Check sheet for the modelled part. Datum: model origin and axes. Units: mm. Face numbers are marked on the shaded views. Round coordinates to 2 decimals unless told otherwise and drop trailing zeros. Write each loop counter-clockwise with the first axis right and the second up, starting at its lowest first coordinate (ties: lowest second). Pieces come first, ordered by that corner, then holes. Notation, with made-up numbers: M 67,4.5 L 122,4.5 A28 ccw 122,35.5 Z; hole C 80.5,65 d7. An arc over 180 degrees is marked long. One line per item, written item: value.
from build123d import *

# Parameters (mm, degrees)
F1_DEPTH = 100
F2_R     = 7.5
F3_DEPTH = 10
F4_R     = 4
F6_DEPTH = 25


with BuildPart() as f1:
    # F0 (on Top) → F1 (new body)
    with BuildSketch(Plane.XY):
        Polygon((25.9807621135, -45), (25.9807621135, 45), (-51.9615242271, 0), align=None)
    extrude(amount=F1_DEPTH)

    # F2 (on face) → F3 (cut)
    with BuildSketch(Plane.YZ.offset(25.9807621135)):
        with Locations((-30, 80)):
            Circle(F2_R)
        with Locations((30, 80)):
            Circle(F2_R)
    extrude(amount=-F3_DEPTH, mode=Mode.SUBTRACT)

    # F4
    f4_edges = [f1.edges().sort_by_distance(p)[0] for p in [
        (25.980762, -45, 50),
        (25.980762, 45, 50),
        (-51.961524, 0, 50),
        (-12.990381, -22.5, 100),
        (-12.990381, 22.5, 100),
        (25.980762, 0, 100),
        (-12.990381, -22.5, 0),
        (25.980762, 0, 0),
        (-12.990381, 22.5, 0),
    ]]
    fillet(f4_edges, radius=F4_R)

    # F5 (on face) → F6 (cut)
    with BuildSketch(Plane(origin=(0, 0, 0), x_dir=(1, 0, 0), z_dir=(0, 0, -1))):
        with BuildLine():
            Line((12.2403810568, -21.2009618943), (9.7403810568, -16.8708348754))
            ThreePointArc((9.7403810568, -16.8708348754), (8.8253175473, -20.2858983849), (12.2403810568, -21.2009618943))
        make_face()
        with BuildLine():
            ThreePointArc((13.4903810568, -19.0358983849), (12.2403810568, -16.8708348754), (9.7403810568, -16.8708348754))
            Line((9.7403810568, -16.8708348754), (12.2403810568, -21.2009618943))
            ThreePointArc((12.2403810568, -21.2009618943), (13.1554445662, -20.2858983849), (13.4903810568, -19.0358983849))
        make_face()
        with BuildLine():
            ThreePointArc((-24.4807621135, 0), (-21.9807621135, -2.5), (-19.4807621135, 0))
            Line((-19.4807621135, 0), (-24.4807621135, 0))
        make_face()
        with BuildLine():
            Line((-24.4807621135, 0), (-19.4807621135, 0))
            ThreePointArc((-19.4807621135, 0), (-21.9807621135, 2.5), (-24.4807621135, 0))
        make_face()
        with BuildLine():
            ThreePointArc((12.2403810568, 21.2009618943), (8.8253175473, 20.2858983849), (9.7403810568, 16.8708348754))
            Line((9.7403810568, 16.8708348754), (12.2403810568, 21.2009618943))
        make_face()
        with BuildLine():
            Line((12.2403810568, 21.2009618943), (9.7403810568, 16.8708348754))
            ThreePointArc((9.7403810568, 16.8708348754), (12.2403810568, 16.8708348754), (13.4903810568, 19.0358983849))
            ThreePointArc((13.4903810568, 19.0358983849), (13.1554445662, 20.2858983849), (12.2403810568, 21.2009618943))
        make_face()
    extrude(amount=-F6_DEPTH, mode=Mode.SUBTRACT)


solid = f1.part
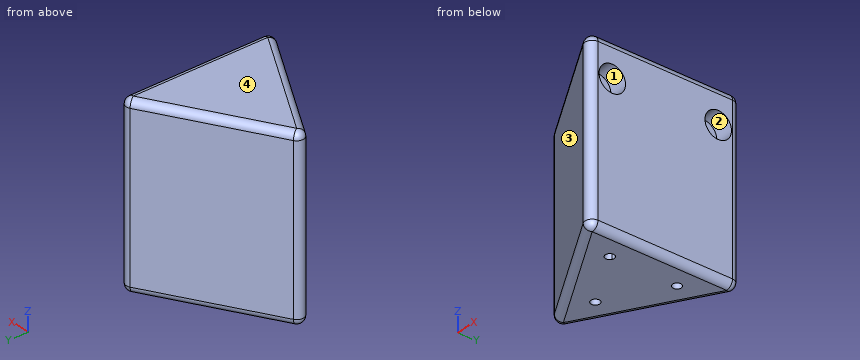
Q1. Scan lines: line 1 (Z direction, x = 18.5, y = 30); line 2 (Z direction, x = 17, y = -35); line 3 (Y direction, x = 20, z = 37). Record each from-to range of solid material in increasing order. Write a range as [from, to].
Completed:
line 1: [0, 72.5], [87.5, 100]
line 2: [0, 74.41], [85.59, 100]
line 3: [-41.55, 41.55]
Q2. Sectioned sample at B-B on z = 80. Enter the section's corners in (x, y).
Completed:
outline: M -45.96,-3.46 L 19.98,-41.54 A4 ccw 25.98,-38.07 L 25.98,-37.5 L 15.98,-37.5 L 15.98,-22.5 L 25.98,-22.5 L 25.98,22.5 L 15.98,22.5 L 15.98,37.5 L 25.98,37.5 L 25.98,38.07 A4 ccw 19.98,41.54 L -45.96,3.46 A4 ccw Z
Q3. Draft check along Z on the marked faces 1, 2, 3 and 4. Enter one of: pulls with the +Z half, pulls with the -Z half, needs draft (parallel to the pull), parting line crosses it, or undercut.
Completed:
face 1: undercut
face 2: undercut
face 3: needs draft
face 4: pulls with the +Z half
Q4. Sectioned sample at A-A on z = 13. Enter the section's corners in (x, y).
Completed:
outline: M -45.96,-3.46 L 19.98,-41.54 A4 ccw 25.98,-38.07 L 25.98,38.07 A4 ccw 19.98,41.54 L -45.96,3.46 A4 ccw Z; hole C -21.98,0 d5; hole C 10.99,-19.04 d5; hole C 10.99,19.04 d5
Q5. Sectioned sample at C-C on z = 37.5. Enter the section's corners in (x, y).
Completed:
outline: M -45.96,-3.46 L 19.98,-41.54 A4 ccw 25.98,-38.07 L 25.98,38.07 A4 ccw 19.98,41.54 L -45.96,3.46 A4 ccw Z
Q6. Depth check by flat-ended pin: P1, Ø8, axis at x = 17.5, z = 87.5, coming from the +Y side; P2, Ø12, axis at y = 30, z = 80, coming from the -X side; P3, Ø1.5, axis at x = 10, y = 18, coming from the -Z side. Enter the tip coordinate at first touch or a pass-through.
Completed:
P1: y = 42.04
P2: x = -10.39
P3: z = 25
